```python
from build123d import *

# Parameters (mm, degrees)
SKETCH_1_W          = 53
SKETCH_1_H          = 20
EXTRUDE_1_DEPTH     = 2
SKETCH_2_W          = 2
SKETCH_2_H          = 20
EXTRUDE_2_DEPTH     = 30
CUT_EXTRUDE_START   = -30
CUT_EXTRUDE_1_DEPTH = 82
SKETCH_4_R          = 1
SKETCH_4_R_2        = 5.25
CUT_EXTRUDE_2_DEPTH = 2
SKETCH_5_R          = 1.3
CUT_EXTRUDE_3_DEPTH = 33


with BuildPart() as part:
    # 草圖1 → 填料-伸長1 (new body)
    with BuildSketch(Plane.XY):
        Rectangle(SKETCH_1_W, SKETCH_1_H)
    extrude(amount=EXTRUDE_1_DEPTH)

    # 草圖2 → 填料-伸長2 (add)
    with BuildSketch(Plane.XY.offset(2)):
        with Locations((-25.5, 0)):
            Rectangle(SKETCH_2_W, SKETCH_2_H)
    extrude_2 = extrude(amount=EXTRUDE_2_DEPTH)

    # 草圖3 → 除料-伸長1 (cut)
    with BuildSketch(Plane(origin=(-24.5, 0, 0), x_dir=(0, 0, -1), z_dir=(1, 0, 0)).offset(CUT_EXTRUDE_START)):
        with BuildLine():
            Line((-32, 10), (-32, 0))
            ThreePointArc((-32, 0), (-29.071067812, 7.071067812), (-22, 10))
            Line((-22, 10), (-32, 10))
        make_face()
        with BuildLine():
            Line((-32, -10), (-22, -10))
            ThreePointArc((-22, -10), (-29.071067812, -7.071067812), (-32, 0))
            Line((-32, 0), (-32, -10))
        make_face()
    cut_extrude_1 = extrude(amount=CUT_EXTRUDE_1_DEPTH, mode=Mode.SUBTRACT)

    # 草圖4 → 除料-伸長2 (cut)
    with BuildSketch(Plane.ZY.offset(26.5)):
        with Locations((29, 0)):
            Circle(SKETCH_4_R)
        with Locations((26.949747468, -4.949747468)):
            Circle(SKETCH_4_R)
        with Locations((22, -7)):
            Circle(SKETCH_4_R)
        with Locations((17.050252532, -4.949747468)):
            Circle(SKETCH_4_R)
        with Locations((15, 0)):
            Circle(SKETCH_4_R)
        with Locations((17.050252532, 4.949747468)):
            Circle(SKETCH_4_R)
        with Locations((22, 7)):
            Circle(SKETCH_4_R)
        with Locations((26.949747468, 4.949747468)):
            Circle(SKETCH_4_R)
        with Locations((22, 0)):
            Circle(SKETCH_4_R_2)
    cut_extrude_2 = extrude(amount=-CUT_EXTRUDE_2_DEPTH, mode=Mode.SUBTRACT)

    # 鏡射1: 填料-伸長2, 除料-伸長1, 除料-伸長2 across plane
    add(extrude_2.mirror(Plane(origin=(0, 0, 0), x_dir=(0, 0, 1), z_dir=(1, 0, 0))))
    add(cut_extrude_1.mirror(Plane(origin=(0, 0, 0), x_dir=(0, 0, 1), z_dir=(1, 0, 0))), mode=Mode.SUBTRACT)
    add(cut_extrude_2.mirror(Plane(origin=(0, 0, 0), x_dir=(0, 0, 1), z_dir=(1, 0, 0))), mode=Mode.SUBTRACT)

    # 草圖5 → 除料-伸長3 (cut, through all)
    with BuildSketch(Plane(origin=(0, 0, 0), x_dir=(-1, 0, 0), z_dir=(0, 0, -1))):
        with Locations((-7, 0)):
            Circle(SKETCH_5_R)
        with Locations((-4.949747468, 4.949747468)):
            Circle(SKETCH_5_R)
        with Locations((0, 7)):
            Circle(SKETCH_5_R)
        with Locations((4.949747468, 4.949747468)):
            Circle(SKETCH_5_R)
        with Locations((7, 0)):
            Circle(SKETCH_5_R)
        with Locations((4.949747468, -4.949747468)):
            Circle(SKETCH_5_R)
        with Locations((0, -7)):
            Circle(SKETCH_5_R)
        with Locations((-4.949747468, -4.949747468)):
            Circle(SKETCH_5_R)
    extrude(amount=-CUT_EXTRUDE_3_DEPTH, mode=Mode.SUBTRACT)


solid = part.part
```
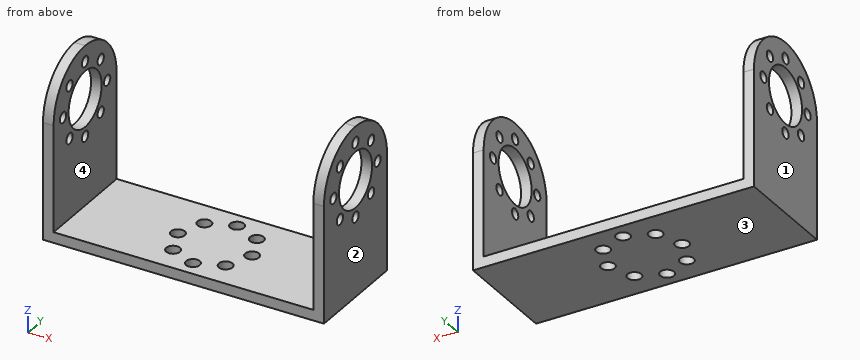
The listing builds one solid part. Answer for the finished solid, in the listing's coordinates (mm). Face numbers are marked on the shaded views. Round coordinates to 2 decimals unless told otherwise and drop trailing zeros. Order: outer loops, then holes, each group sorted by start corner. A loop starts at its lowest first (then second) coordinate and runs counter-clockwise, first axis right, second up. Notation, with made-up numbers: (-32.5, 26.25) -> (-19.5, 26.25) arc R22 cw to (-19.5, 41.25) -> close; hole circle Ø7 at (-5.75, -7). An arc over 180 degrees is marked (long way). Answer as CSV lines item,"result".
Q1. A cutting plane is placed at A-A on x = 0. Determine the outline of the cut face in (y, z).
Computed values:
outline,"(-10, 0) -> (-8.3, 0) -> (-8.3, 2) -> (-10, 2) -> close; (-5.7, 0) -> (5.7, 0) -> (5.7, 2) -> (-5.7, 2) -> close; (8.3, 0) -> (10, 0) -> (10, 2) -> (8.3, 2) -> close"
Q2. A cutting plane is placed at C-C on z = 15. Determine the outline of the cut face in (x, y), plus the area to 3 significant figures.
Computed values:
outline,"(-26.5, -10) -> (-24.5, -10) -> (-24.5, -1) -> (-26.5, -1) -> close; (-26.5, 1) -> (-24.5, 1) -> (-24.5, 10) -> (-26.5, 10) -> close; (24.5, -10) -> (26.5, -10) -> (26.5, -1) -> (24.5, -1) -> close; (24.5, 1) -> (26.5, 1) -> (26.5, 10) -> (24.5, 10) -> close"
area,"72.0 mm^2"
Q3. A cutting plane is placed at D-D on z = 7.5. Determine the outline of the cut face in (x, y).
Computed values:
outline,"(-26.5, -10) -> (-24.5, -10) -> (-24.5, 10) -> (-26.5, 10) -> close; (24.5, -10) -> (26.5, -10) -> (26.5, 10) -> (24.5, 10) -> close"
Q4. For a pull along X with two mould halves and no side action, classify the marked faces 1, 2, 3 and 4 as +X half, -X half, draft (parallel to the pull), parting line (faces both ways), or undercut.
Computed values:
face 1,"-X half"
face 2,"+X half"
face 3,"draft"
face 4,"undercut"
Q5. Consider line 1 (Y direction, x = -25.1, z = 22); line 2 (X direction, y = 4, z = 30); line 3 (Y direction, x = 7, z = 1). Determine where each line is inside the solid, lowest interval first. Write a range as from..to.
Computed values:
line 1,"y = -10..-8, -6..-5.25, 5.25..6, 8..10"
line 2,"x = -26.5..-24.5, 24.5..26.5"
line 3,"y = -10..-1.3, 1.3..10"
Q6. A cutting plane is placed at B-B on x = -7. Determine the outline of the cut face in (y, z).
Computed values:
outline,"(-10, 0) -> (-1.3, 0) -> (-1.3, 2) -> (-10, 2) -> close; (1.3, 0) -> (10, 0) -> (10, 2) -> (1.3, 2) -> close"
Q7. Given pin 1 (4 mm diameter, centred on x = -7, y = 0, fed in from +Z); pin 2 (1.6 mm diameter, centred on x = -4.95, y = 4.95, fed in from +Z), each flat-ended and moving along its own axis, determine where each tip first touches the part or whether it passes through.
Computed values:
pin 1,"stops at z = 2"
pin 2,"passes through"
